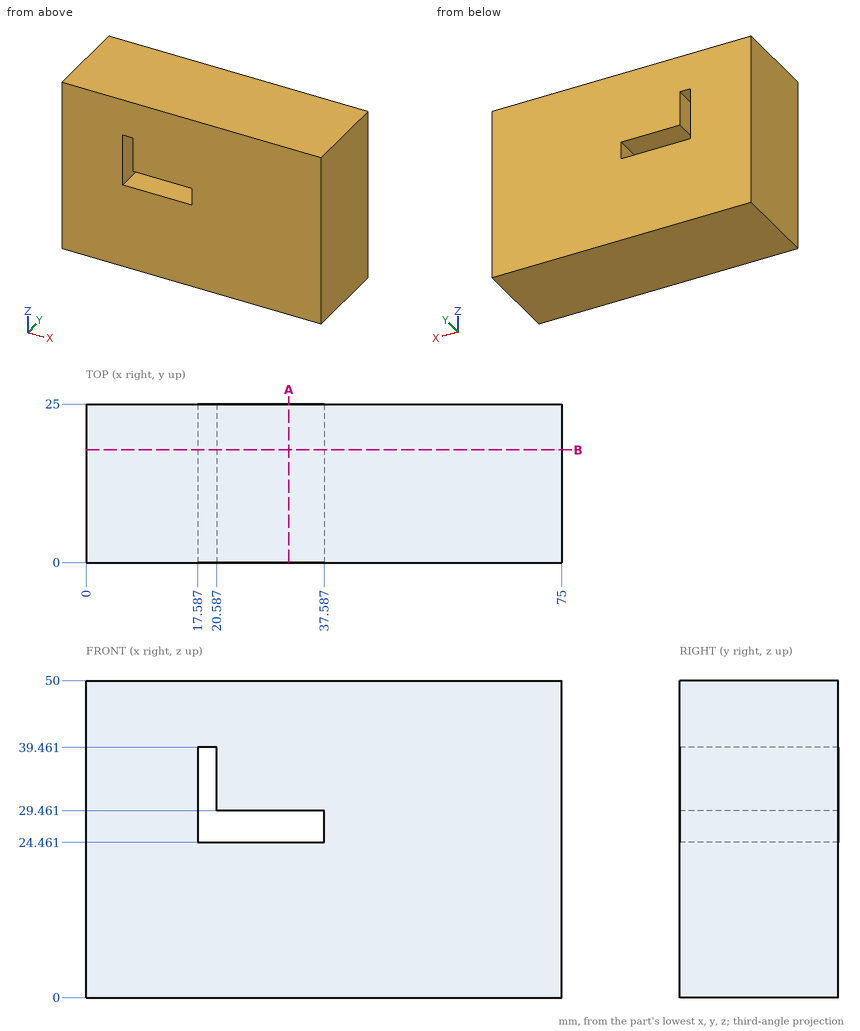
Here's the drawing with two shaded views (mm, measured from the low corner). I have some questions. Round coordinates to 2 decimals unless told otherwise and drop trailing zeros. Order: outer loops, then holes, each group sorted by start corner. A loop starts at its lowest first (then second) coordinate and runs counter-clockwise, first axis right, second up. Notation, with made-up numbers: M 51,28.25 L 104,28.25 A11 ccw 104,33.25 Z; hole C 51.25,-9.75 d7. An arc over 180 degrees is marked long. Answer in a Markdown table with one row per item.
Item 1: Imagine slicing it at B-B, the plane y = 17.75. Write out the boundary of the cut face in (x, z), and give its area (3 significant figures).
A:
| item | result |
|---|---|
| outline | M 0,0 L 75,0 L 75,50 L 0,50 Z; hole M 17.59,24.46 L 37.59,24.46 L 37.59,29.46 L 20.59,29.46 L 20.59,39.46 L 17.59,39.46 Z |
| area | 3,620 mm2 |
Item 2: I'm going to push a flat-ended pin straight in: pin 1 (2 mm diameter, centred on x = 35.5, z = 25.5, fed in from +Y). Where does the tip first touch, or does it pass through?
A:
| item | result |
|---|---|
| pin 1 | passes through |
Item 3: If I drill on L1, parallel to Z at x = 23, y = 2; L2, parallel to X at y = 13.25, z = 37.5; L3, parallel to X at y = 18, z = 26, over which ranges is the centre line in solid material (lowest first)? Write a range as from..to.
A:
| item | result |
|---|---|
| L1 | z = 0..24.46, 29.46..50 |
| L2 | x = 0..17.59, 20.59..75 |
| L3 | x = 0..17.59, 37.59..75 |
Item 4: Imagine slicing it at A-A, the plane x = 32. Write out the boundary of the cut face in (y, z), and give its area (4 significant figures).
A:
| item | result |
|---|---|
| outline | M 0,0 L 25,0 L 25,24.46 L 0,24.46 Z; M 0,29.46 L 25,29.46 L 25,50 L 0,50 Z |
| area | 1,125 mm2 |
